from build123d import *

# Parameters (mm, degrees)
F1_DEPTH = 152.4
F2_R     = 7.874
F3_R     = 3.302


with BuildPart() as f1:
    # F0 (on Front) → F1 (new body, symmetric)
    with BuildSketch(Plane.XZ):
        Polygon((-88.9, 0), (0, 0), (88.9, 0), (88.9, 53.086), (83.566, 53.086), (75.692, 5.334), (0, 5.334), (-75.692, 5.334), (-83.566, 53.086), (-88.9, 53.086), align=None)
    extrude(amount=F1_DEPTH, both=True)

    # F2
    f2_edges = [f1.edges().sort_by_distance(p)[0] for p in [
        (-75.692, 0, 5.334),
        (75.692, 0, 5.334),
    ]]
    fillet(f2_edges, radius=F2_R)

    # F3
    f3_edges = [f1.edges().sort_by_distance(p)[0] for p in [
        (83.566, 0, 53.086),
        (-83.566, 0, 53.086),
    ]]
    fillet(f3_edges, radius=F3_R)


solid = f1.part
Can you work these out from the model? Positions are in its coordinate system, mm. A direction names the side the tool comes from. Give positions to 0.01 mm unless a question says otherwise; leave off trailing zeros. Order: outer loops, then holes, each group sorted by start corner. A loop starts at its lowest first (then second) coordinate and runs counter-clockwise, first axis right, second up. Notation, with made-up numbers: M 69.5,-18.75 L 86.5,-18.75 A27 ccw 86.5,9.25 Z; hole C 38,20.5 d9. An arc over 180 degrees is marked long. One line per item, written item: value.
Item 1: For pin 1 (5 mm diameter, centred on x = 67.5, y = 34, fed in from +Z); pin 2 (3 mm diameter, centred on x = -15.5, y = -41, fed in from +Z); pin 3 (8 mm diameter, centred on x = 21, z = 13, fed in from -Y), each with a flat end and sliding along its axis, tell me the tip position at first contact or that it passes through.
Verdict:
pin 1: z = 5.4
pin 2: z = 5.33
pin 3: through
Item 2: Please list where these lines run through material, in increasing order: line 1 (Z direction, x = -3, y = 97); line 2 (X direction, y = 31.5, z = 25); line 3 (X direction, y = 81, z = 25.5).
Verdict:
line 1: 0 to 5.33
line 2: -88.9 to -78.93, 78.93 to 88.9
line 3: -88.9 to -79.02, 79.02 to 88.9
Item 3: If we section it at A-A on y = 126: Write out the boundary of the cut face in (x, z).
Verdict:
outline: M -88.9,0 L 88.9,0 L 88.9,53.09 L 86.37,53.09 A3.3 ccw 83.11,50.32 L 76.78,11.93 A7.87 cw 69.01,5.33 L -69.01,5.33 A7.87 cw -76.78,11.93 L -83.11,50.32 A3.3 ccw -86.37,53.09 L -88.9,53.09 Z
Item 4: If we section it at B-B on z = 19.5: Write out the boundary of the cut face in (x, y).
Verdict:
outline: M -88.9,-152.4 L -78.03,-152.4 L -78.03,152.4 L -88.9,152.4 Z; M 78.03,-152.4 L 88.9,-152.4 L 88.9,152.4 L 78.03,152.4 Z
Item 5: For faces 1 (the face through (88.9, -2, 26)), 2 (the face through (74.045, -2.134, 7.154)), which set-ups out of +Z, -Z, +X, -X, +Y, -Y let a thin tool reach every point of the face, with its end or its side?
Verdict:
face 1: +Z, -Z, +X, +Y, -Y
face 2: +Z, +Y, -Y
Item 6: If we section it at C-C on x = 50.5: Write out the boundary of the cut face in (y, z), and give its area (3 significant figures).
Verdict:
outline: M -152.4,0 L 152.4,0 L 152.4,5.33 L -152.4,5.33 Z
area: 1,630 mm2
Item 7: If we section it at D-D on z = 44: Write out the boundary of the cut face in (x, y).
Verdict:
outline: M -88.9,-152.4 L -82.07,-152.4 L -82.07,152.4 L -88.9,152.4 Z; M 82.07,-152.4 L 88.9,-152.4 L 88.9,152.4 L 82.07,152.4 Z
